from build123d import *

# Parameters (mm, degrees)
BOSS_EXTRUDE2_DEPTH   = 14
BOSS_EXTRUDE2_2_DEPTH = 14
BOSS_EXTRUDE3_DEPTH   = 1
BOSS_EXTRUDE6_DEPTH   = 159.193
BOSS_EXTRUDE7_DEPTH   = 4.707
BOSS_EXTRUDE8_DEPTH   = 9.5
BOSS_EXTRUDE9_DEPTH   = 7.107
BOSS_EXTRUDE10_DEPTH  = 14.207
SKETCH7_W             = 16
SKETCH7_H             = 8.5
CUT_EXTRUDE1_DEPTH    = 4
FILLET1_R             = 3
FILLET2_R             = 3
SKETCH8_W             = 2
SKETCH8_H             = 42.28
BOSS_EXTRUDE11_DEPTH  = 7
SKETCH9_W             = 16
SKETCH9_H             = 5.5
BOSS_EXTRUDE12_DEPTH  = 3


with BuildPart() as part:
    # Sketch3 → Boss-Extrude2 (new body)
    with BuildSketch(Plane(origin=(0, 0, 0), x_dir=(1, 0, 0), z_dir=(0, 1, 0))):
        Polygon((0, 78.28), (0, 0), (-163.3, 0), (-163.3, -3), (3, -3), (3, 78.28), align=None)
    extrude(amount=BOSS_EXTRUDE2_DEPTH)

    # Sketch3<3> → Boss-Extrude3 (add)
    with BuildSketch(Plane(origin=(0, 0, 0), x_dir=(1, 0, 0), z_dir=(0, 1, 0))):
        Polygon((-163.3, 19.1), (-163.3, -3), (3, -3), (3, 78.28), (0, 78.28), (0, 114.28), (-156.193, 114.28), (-156.193, 76.28), (-165.693, 76.28), (-165.693, 57.2), (-160.9, 57.2), (-160.9, 38), (-170.4, 38), (-170.4, 19.1), align=None)
    extrude(amount=-BOSS_EXTRUDE3_DEPTH)



with BuildPart() as body_2:
    # Sketch3 → Boss-Extrude2 2 (new body)
    with BuildSketch(Plane(origin=(0, 0, 0), x_dir=(1, 0, 0), z_dir=(0, 1, 0))):
        Polygon((0, 114.28), (0, 94.28), (3, 94.28), (3, 117.28), (-156.193, 117.28), (-156.193, 114.28), align=None)
    extrude(amount=BOSS_EXTRUDE2_2_DEPTH)


with BuildPart() as part_1:
    add(part.part)

    add(body_2.part)  # Boss-Extrude6 merges body 2
    # Sketch4 → Boss-Extrude6 (add)
    with BuildSketch(Plane(origin=(3, 0, 0), x_dir=(0, 0, -1), z_dir=(1, 0, 0))):
        Polygon((-3, -1), (117.28, -7.303607692), (117.28, 0), (-3, 0), align=None)
    extrude(amount=-BOSS_EXTRUDE6_DEPTH)

    # Sketch5 → Boss-Extrude7 (add)
    with BuildSketch(Plane.ZY.offset(156.193)):
        Polygon((-38, 0), (-57.2, 0), (-57.2, -4.154948313), (-38, -3.148718951), align=None)
    extrude(amount=BOSS_EXTRUDE7_DEPTH)

    # Sketch5<4> → Boss-Extrude8 (add)
    with BuildSketch(Plane.ZY.offset(156.193)):
        Polygon((-57.2, 0), (-76.28, 0), (-76.28, -5.154888742), (-57.2, -4.154948313), align=None)
    extrude(amount=BOSS_EXTRUDE8_DEPTH)

    # Sketch5 again → Boss-Extrude9 (add)
    with BuildSketch(Plane.ZY.offset(156.193)):
        Polygon((3, -1), (-19.1, -1), (-19.1, -2.158211922), align=None)
    extrude(amount=BOSS_EXTRUDE9_DEPTH)

    # Sketch5<6> → Boss-Extrude10 (add)
    with BuildSketch(Plane.ZY.offset(156.193)):
        Polygon((-19.1, -1), (-38, -1), (-38, -3.148718951), (-19.1, -2.158211922), align=None)
    extrude(amount=BOSS_EXTRUDE10_DEPTH)

    # Sketch7 → Cut-Extrude1 (cut)
    with BuildSketch(Plane.ZY):
        with Locations((-28, 4.25)):
            Rectangle(SKETCH7_W, SKETCH7_H)
    extrude(amount=-CUT_EXTRUDE1_DEPTH, mode=Mode.SUBTRACT)

    # Fillet1
    fillet1_edges = [part_1.edges().sort_by_distance(p)[0] for p in [
        (3, 3.348196154, -117.28),
    ]]
    fillet(fillet1_edges, radius=FILLET1_R)

    # Fillet2
    fillet2_edges = [part_1.edges().sort_by_distance(p)[0] for p in [
        (3, 6.5, 3),
    ]]
    fillet(fillet2_edges, radius=FILLET2_R)

    # Sketch8 → Boss-Extrude11 (add)
    with BuildSketch(Plane(origin=(0, 0, 0), x_dir=(1, 0, 0), z_dir=(0, 1, 0))):
        Polygon((-154.193, 112.28), (-2, 112.28), (-2, 94.28), (0, 94.28), (0, 114.28), (-156.193, 114.28), (-156.193, 76.28), (-165.693, 76.28), (-165.693, 57.2), (-160.9, 57.2), (-160.9, 38), (-170.4, 38), (-170.4, 19.1), (-163.3, 19.1), (-163.3, 0), (0, 0), (0, 20), (-2, 20), (-2, 2), (-161.3, 2), (-161.3, 21.1), (-168.4, 21.1), (-168.4, 36), (-158.9, 36), (-158.9, 59.2), (-163.693, 59.2), (-163.693, 74.28), (-154.193, 74.28), align=None)
        with Locations((-1, 57.14)):
            Rectangle(SKETCH8_W, SKETCH8_H)
    extrude(amount=BOSS_EXTRUDE11_DEPTH)

    # Sketch9 → Boss-Extrude12 (add)
    with BuildSketch(Plane.ZY):
        with Locations((-86.28, 11.25)):
            Rectangle(SKETCH9_W, SKETCH9_H)
    extrude(amount=-BOSS_EXTRUDE12_DEPTH)


solid = part_1.part
Input: part model. Units: mm. Frame: model coordinates. A direction names the side the tool comes from. Coordinates: 2 decimals unless noted, no trailing zeros. Write each loop counter-clockwise with the first axis right and the second up, starting at its lowest first coordinate (ties: lowest second). Pieces come first, ordered by that corner, then holes. Notation, with made-up numbers: M 37.25,53.25 L 65.25,53.25 A13 cw 65.25,61.25 Z; hole C -2,63.25 d1. An arc over 180 degrees is marked long. Answer as a JSON object with one key per item and string values. Group by question number.
(1) Ray query, line 1 along X through (y, z) = (4.25, -51); line 2 along Z through (x, y) = (-58.5, 12.75); line 3 along Z through (x, y) = (-109.5, 5.25). Return the intervals inside material, ascending. Write a range as [from, to].
(2) Section D-D on z = -64. Output: boundary loops of the cut face in (x, y), plus the area to 3 significant figures.
(3) Mould query, pull axis Z, two halves, no side actions, for faces 1 (the face through (-83, 7, 3)), 2 (the face through (3, 6, -58)), 3 (the face through (1, 4, -78.28)). Classes: pulls with the +Z half, pulls with the -Z half, needs draft (parallel to the pull), parting line crosses it, or undercut.
(4) Section B-B on z = -84.5. Output: boundary loops of the cut face in (x, y), plus the area to 3 significant figures.
(5) Contact query for flat-ended pins moving along their axis: P1, Ø1, axis at x = -84.5, z = -82, coming from the -Y side; P2, Ø2, axis at x = -168, y = 4.5, coming from the +Z side; P3, Ø12, axis at x = -60, z = -53, coming from the +Y side. Output: stop coordinate, or through.
(6) Set-up query: faces 4 (the face through (-161.3, 3, -11)), 5 (the face through (0, 4, -20)), 6 (the face through (-168.4, 3, -28)), 7 (the face through (-160.9, 1, -48)). Return all of +Z, -Z, +X, -X, +Y, -Y with unobstructed straight access to the full face (end or side cutting, diameter ignored); none if empty.
(7) Section C-C on x = -74. Output: boundary loops of the cut face in (y, z), plus the area to 3 significant figures.
Result set:
{
 "1": {"line 1": "x = [-160.9, -158.9], [-2, 3]", "line 2": "z = [-117.28, -114.28], [0, 3]", "line 3": "z = [-117.28, -112.28], [-2, 3]"},
 "2": {"outline": "M -165.69,-4.51 L 3,-4.51 L 3,14 L 0,14 L 0,7 L -2,7 L -2,0 L -163.69,0 L -163.69,7 L -165.69,7 Z", "area": "831 mm2"},
 "3": {"face 1": "pulls with the +Z half", "face 2": "needs draft", "face 3": "undercut"},
 "4": {"outline": "M -156.19,-5.59 L 3,-5.59 L 3,0 L -154.19,0 L -154.19,7 L -156.19,7 Z; M 0,8.5 L 3,8.5 L 3,14 L 0,14 Z", "area": "920 mm2"},
 "5": {"P1": "stops at y = -5.48", "P2": "stops at z = -19.1", "P3": "stops at y = 0"},
 "6": {"face 4": "+Y", "face 5": "+X", "face 6": "+X, +Y", "face 7": "-X, +Y, -Y"},
 "7": {"outline": "M -7.3,-117.28 L 14,-117.28 L 14,-114.28 L 7,-114.28 L 7,-112.28 L 0,-112.28 L 0,-2 L 7,-2 L 7,0 L 14,0 L 14,3 L -1,3 Z", "area": "611 mm2"}
}
